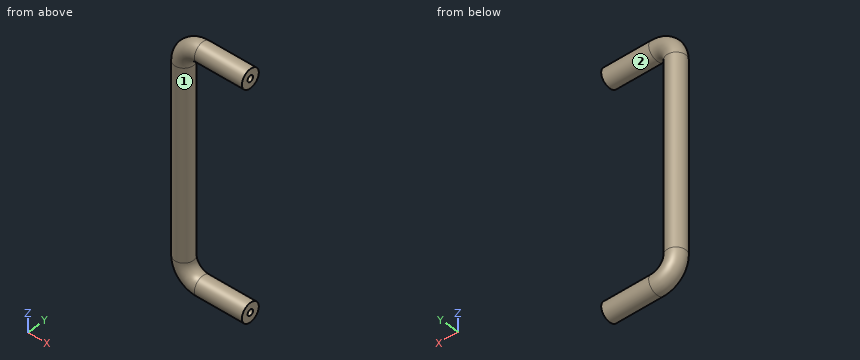
Autodesk Inventor part; units mm, degrees
ref_plane "YZ Plane" through (0, 0, 0) normal (1, 0, 0) x (0, 1, 0)
ref_plane "XZ Plane" through (0, 0, 0) normal (0, 1, 0) x (-1, 0, 0)
ref_plane "XY Plane" through (0, 0, 0) normal (0, 0, 1) x (1, 0, 0)
sketch "Skizze1" plane through (0, 0, 0) normal (0, 1, 0) x (-1, 0, 0)
  line L0 (0, 0) -> (25, 0)
  line L1 (35, -10) -> (35, -110)
  line L2 (25, -120) -> (0, -120)
  arc A0 (35, -10) -> (25, 0) centre (25, -10) ccw
  arc A1 (25, -120) -> (35, -110) centre (25, -110) ccw
  point P0 (35, 0)
  point P1 (35, -120)
  dimension "d0" = 35
  dimension "d1" = 120
  dimension "d2" = 10
sketch "Skizze2" plane through (0, 0, 0) normal (1, 0, 0) x (0, 1, 0)
  circle A0 centre (0, 0) radius 5
  dimension "d3" = 10
sweep "Sweeping1" add profiles "Skizze2" path "Skizze1"
sketch "Skizze3" plane through (0, 0, 0) normal (1, 0, 0) x (0, 0, -1)
  circle A0 centre (0, 0) radius 5
  point P0 (120, 0)
hole "Bohrung1" at (0, 0, 0) at (0, 0, -120) direction (-1, 0, 0) diameter 3.242 depth 11.8 tip angle 118
properties part number "Blechgriff"
Build history of the part. All positions in model axes, mm. Face numbers are marked on the shaded views. A direction names the side the tool comes from. Give positions to 0.01 mm unless a question says otherwise; leave off trailing zeros. Order: outer loops, then holes, each group sorted by start corner. A loop starts at its lowest first (then second) coordinate and runs counter-clockwise, first axis right, second up. Notation, with made-up numbers: M 64,48 L 68,48 A15 cw 68,54 Z; hole C 80.5,13.5 d3. An arc over 180 degrees is marked long. Use one line per item in the form item = value.
Q1. Slice it at C-C, the plane y = -3.75. Write the cut outline in (x, z), and give its area (3 significant figures).
Conclusion:
outline = M -38.31,-110 A13.31 ccw -25,-123.31 L 0,-123.31 L 0,-116.69 L -25,-116.69 A6.69 cw -31.69,-110 L -31.69,-10 A6.69 cw -25,-3.31 L 0,-3.31 L 0,3.31 L -25,3.31 A13.31 ccw -38.31,-10 Z
area = 1,200 mm2
Q2. Pin check, flat tips, straight feed: P1, Ø4, axis at y = 0, z = 0, coming from the +X side; P2, Ø12, axis at x = -26.5, z = -97, coming from the -Y side; P3, Ø3, axis at y = 0, z = -120, coming from the -X side; P4, Ø1, axis at y = -3.5, z = -89.5, coming from the +X side. Stop position of each tip, or through.
Conclusion:
P1 = 0
P2 = -4.33
P3 = -37.36
P4 = -31
Q3. Slice it at B-B, the plane z = -42. Write the cut outline in (x, y), and give its area (3 significant figures).
Conclusion:
outline = C -35,0 d10
area = 78.5 mm2
Q4. Slice it at A-A, the plane x = -8. Write the cut outline in (y, z), and give its area (3 significant figures).
Conclusion:
outline = C 0,-120 d10; C 0,0 d10; hole C 0,-120 d3.24; hole C 0,0 d3.24
area = 141 mm2
Q5. Wall check: probe 1 along Z at (x, y) = (-7.25, 0); probe 2 along Y at (x, z) = (-2.75, 0); probe 3 along Z at (x, y) = (-17.5, 3). Give the ranges that are in metal, low to high.
Conclusion:
probe_1 = -125 to -121.62, -118.38 to -115, -5 to -1.62, 1.62 to 5
probe_2 = -5 to -1.62, 1.62 to 5
probe_3 = -124 to -116, -4 to 4
Q6. Which spindle directions (+Z, -Z, +X, -X, +Y, -Y) get a long thin tool onto all of the face, cutting with end or side? Do the marked faces 1 and 2. Say none if no direction does.
Conclusion:
face_1 = none
face_2 = +X
